Work out the finished part from the listing and answer in its coordinate system (mm). A direction names the side the tool comes from. Give positions to 0.01 mm unless a question says otherwise; leave off trailing zeros. Write each loop counter-clockwise with the first axis right and the second up, starting at its lowest first coordinate (ties: lowest second). Pieces come first, ordered by that corner, then holes. Notation, with made-up numbers: (-16, 35) -> (21, 35) arc R32 cw to (21, 67) -> close; hole circle Ø11 at (76.25, 79.5). An arc over 180 degrees is marked (long way). Use a Markdown table: item, result. Add a question column.
Q1. Section D-D, the plane z = -3 is taken. Give the vertices of the cut face in (x, y).
Q2. Section A-A, the plane z = -7 is taken. Give the vertices of the cut face in (x, y) (3 decimals).
Q3. Each of these flat-tipped pins is pushed along its axis until it touches: pin 1 Ø2 at (x, z) = (-3, -10) entering from -Y; pin 2 Ø2 at (y, z) = (5.5, -3.5) entering from -X; pin 3 Ø3 at (x, z) = (12.5, -7.5) entering from +Y; pin 4 Ø0.5 at (x, z) = (-3, -10) entering from +Y. Where does it stop, or does it pass through?
Q4. For a pull along Z with two mould halves and no side action, classify faces 5 (the face through (34, 36, -7)), 6 (the face through (2, 29, 0)), 7 (the face through (36, 6, -2)) as pulls with the +Z half, pulls with the -Z half, needs draft (parallel to the pull), parting line crosses it, or undercut.
Q5. Consider line 1 (X direction, y = 54.5, z = -8); line 2 (X direction, y = 61.5, z = -2.25); line 3 (Z direction, x = 32.5, y = 42). Determine where each line is inside the solid, lowest interval first.
Q6. For faces 1 (the face through (2.3, 9.07, -3.23)), 2 (the face through (-0.57, 47.5, -10.18)), 3 (the face through (9.275, 1, -7)), 4 (the face through (1, 6, -2)), determine the directions among +Z, -Z, +X, -X, +Y, -Y from which every point of the face is accessible in a straight line to the end or side of a thin tool.
Q7. Section C-C, the plane y = 16 is taken. Give the vertices of the cut face in (x, z), plus the area to 3 significant figures.
Q8. Section B-B, the plane x = 10 is taken. Give the vertices of the cut face in (y, z).
from build123d import *

# Parameters (mm, degrees)
SKETCH1_W           = 37
SKETCH1_H           = 11.7
BOSS_EXTRUDE1_DEPTH = 69
CUT_EXTRUDE1_DEPTH  = 67
SKETCH3_W           = 20
SKETCH3_H           = 5.9
CUT_EXTRUDE2_DEPTH  = 67
SKETCH4_R           = 1.9
BOSS_EXTRUDE2_DEPTH = 3
FILLET1_R           = 2
SKETCH5_W           = 3.5
SKETCH5_H           = 9
CUT_EXTRUDE3_DEPTH  = 40
BOSS_EXTRUDE3_START = 0.5
BOSS_EXTRUDE3_DEPTH = 2.5


with BuildPart() as part:
    # Sketch1 → Boss-Extrude1 (new body)
    with BuildSketch(Plane(origin=(0, 0, 0), x_dir=(1, 0, 0), z_dir=(0, 1, 0))):
        with Locations((18.5, 5.85)):
            Rectangle(SKETCH1_W, SKETCH1_H)
    extrude(amount=BOSS_EXTRUDE1_DEPTH)

    # Sketch2 → Cut-Extrude1 (cut)
    with BuildSketch(Plane(origin=(0, 69, 0), x_dir=(1, 0, 0), z_dir=(0, 1, 0))):
        Polygon((3, 0), (3, 2), (2, 2), (2, 3.8), (3, 3.8), (3, 9.7), (34, 9.7), (34, 3.8), (35, 3.8), (35, 2), (34, 2), (34, 0), align=None)
    extrude(amount=-CUT_EXTRUDE1_DEPTH, mode=Mode.SUBTRACT)

    # Sketch3 → Cut-Extrude2 (cut)
    with BuildSketch(Plane(origin=(0, 2, 0), x_dir=(1, 0, 0), z_dir=(0, 1, 0))):
        with Locations((19.275, 6.75)):
            Rectangle(SKETCH3_W, SKETCH3_H)
    extrude(amount=-CUT_EXTRUDE2_DEPTH, mode=Mode.SUBTRACT)

    # Sketch4 → Boss-Extrude2 (add)
    # profile 1 of 2: a face of its own
    with BuildSketch(Plane(origin=(48.7, 0, -11.7), x_dir=(-1, 0, 0), z_dir=(0, 0, -1))):
        with BuildLine():
            Line((48.7, 55.9), (52.5, 55.9))
            ThreePointArc((52.5, 55.9), (56.4, 52), (52.5, 48.1))
            Line((52.5, 48.1), (48.7, 48.1))
            Line((48.7, 48.1), (48.7, 55.9))
        make_face()
        with Locations((52.5, 52)):
            Circle(SKETCH4_R, mode=Mode.SUBTRACT)
    # profile 2 of 2: a face of its own
    with BuildSketch(Plane(origin=(48.7, 0, -11.7), x_dir=(-1, 0, 0), z_dir=(0, 0, -1))):
        with BuildLine():
            Line((48.7, 19.9), (52.5, 19.9))
            ThreePointArc((52.5, 19.9), (56.4, 16), (52.5, 12.1))
            Line((52.5, 12.1), (48.7, 12.1))
            Line((48.7, 12.1), (48.7, 19.9))
        make_face()
        with Locations((52.5, 16)):
            Circle(SKETCH4_R, mode=Mode.SUBTRACT)
    extrude(amount=-BOSS_EXTRUDE2_DEPTH)

    # Fillet1
    fillet1_edges = [part.edges().sort_by_distance(p)[0] for p in [
        (0, 48.1, -10.2),
        (0, 55.9, -10.2),
        (0, 12.1, -10.2),
        (0, 19.9, -10.2),
    ]]
    fillet(fillet1_edges, radius=FILLET1_R)

    # Sketch5 → Cut-Extrude3 (cut)
    with BuildSketch(Plane(origin=(37, 0, 0), x_dir=(0, 0, -1), z_dir=(1, 0, 0))):
        with Locations((3.25, 6.5)):
            Rectangle(SKETCH5_W, SKETCH5_H)
    extrude(amount=-CUT_EXTRUDE3_DEPTH, mode=Mode.SUBTRACT)

    # Sketch6 → Boss-Extrude3 (add)
    with BuildSketch(Plane(origin=(0, 0, -1.5), x_dir=(-1, 0, 0), z_dir=(0, 0, -1)).offset(BOSS_EXTRUDE3_START)):
        with BuildLine():
            Line((0, 2), (0, 9.5))
            Line((0, 9.5), (-1.25, 9.5))
            ThreePointArc((-1.25, 9.5), (-2.310660172, 9.060660172), (-2.75, 8))
            Line((-2.75, 8), (-2.75, 7.5))
            ThreePointArc((-2.75, 7.5), (-2.457106781, 6.792893219), (-1.75, 6.5))
            Line((-1.75, 6.5), (-1.75, 2))
            Line((-1.75, 2), (0, 2))
        make_face()
    boss_extrude3 = extrude(amount=BOSS_EXTRUDE3_DEPTH)

    # Mirror1: Boss-Extrude3 across plane
    add(boss_extrude3.mirror(Plane.ZY.offset(-18.5)))


solid = part.part
Result set:
| question | item | result |
|---|---|---|
| 1 | outline | (0, 0) -> (37, 0) -> (37, 9.5) -> (35.75, 9.5) arc R1.5 ccw to (34.25, 8) -> (34.25, 7.5) arc R1 ccw to (35.25, 6.5) -> (35.25, 2) -> (1.75, 2) -> (1.75, 6.5) arc R1 ccw to (2.75, 7.5) -> (2.75, 8) arc R1.5 ccw to (1.25, 9.5) -> (0, 9.5) -> close; (0, 11) -> (2, 11) -> (2, 69) -> (0, 69) -> close; (35, 11) -> (37, 11) -> (37, 69) -> (35, 69) -> close |
| 2 | outline | (0, 0) -> (9.275, 0) -> (9.275, 2) -> (3, 2) -> (3, 69) -> (0, 69) -> close; (29.275, 0) -> (37, 0) -> (37, 69) -> (34, 69) -> (34, 2) -> (29.275, 2) -> close |
| 3 | pin 1 | stops at y = 12.1 |
| 3 | pin 2 | stops at x = 0 |
| 3 | pin 3 | passes through |
| 3 | pin 4 | stops at y = 55.9 |
| 4 | face 5 | needs draft |
| 4 | face 6 | pulls with the +Z half |
| 4 | face 7 | undercut |
| 5 | line 1 | x = 0 to 3, 34 to 37 |
| 5 | line 2 | x = 0 to 2, 35 to 37 |
| 5 | line 3 | z = -11.7 to -9.7 |
| 6 | face 1 | none |
| 6 | face 2 | +Z, -Z, -X |
| 6 | face 3 | +Y, -Y |
| 6 | face 4 | +X, -X |
| 7 | outline | (-7.7, -11.7) -> (-5.7, -11.7) -> (-5.7, -8.7) -> (-7.7, -8.7) -> close; (-1.9, -11.7) -> (37, -11.7) -> (37, 0) -> (34, 0) -> (34, -2) -> (35, -2) -> (35, -3.8) -> (34, -3.8) -> (34, -9.7) -> (3, -9.7) -> (3, -3.8) -> (2, -3.8) -> (2, -2) -> (3, -2) -> (3, 0) -> (0, 0) -> (0, -8.7) -> (-1.9, -8.7) -> close |
| 7 | area | 140 mm2 |
| 8 | outline | (0, -11.7) -> (69, -11.7) -> (69, -9.7) -> (0, -9.7) -> close; (0, -3.8) -> (2, -3.8) -> (2, 0) -> (0, 0) -> close |
